Design review of the part built by this model. Coordinates are the model's own, in mm. A direction names the side the tool comes from. Coordinates: 2 decimals unless noted, no trailing zeros. Write each loop counter-clockwise with the first axis right and the second up, starting at its lowest first coordinate (ties: lowest second). Pieces come first, ordered by that corner, then holes. Notation, with made-up numbers: M 81.5,-28.75 L 123.5,-28.75 A35 ccw 123.5,9.25 Z; hole C 81.5,-20 d9. An arc over 180 degrees is marked long. Write item = value, one per line.
```python
from build123d import *

# Parameters (mm, degrees)
ESBO_O1_R                = 15.19
RESSALTO_EXTRUS_O1_DEPTH = 17.37
RESSALTO_EXTRUS_O1_DRAFT = -10
ESBO_O2_R                = 5
CORTE_EXTRUS_O1_DEPTH    = 7
ESBO_O3_R                = 3
CORTE_EXTRUS_O2_DEPTH    = 24.853911629
FILETE1_R                = 2


with BuildPart() as part:
    # Esboço1 → Ressalto-extrusão1 (with draft: the straight prism first)
    with BuildSketch(Plane(origin=(0, 0, 0), x_dir=(1, 0, 0), z_dir=(0, 1, 0))):
        Circle(ESBO_O1_R)
    extrude(amount=-RESSALTO_EXTRUS_O1_DEPTH)
    # Ressalto-extrusão1: the draft: its side faces are tilted about the plane it starts from
    ressalto_extrus_o1_sides = [part.faces().sort_by_distance(p)[0] for p in [
        (-15.19, -8.685, 0),
    ]]
    draft(ressalto_extrus_o1_sides, Plane(origin=(0, 0, 0), x_dir=(1, 0, 0), z_dir=(0, 1, 0)), RESSALTO_EXTRUS_O1_DRAFT)

    # Esboço2 → Corte-extrusão1 (cut)
    with BuildSketch(Plane.XZ.offset(17.37)):
        with Locations(Location((0, 0, 0), (0, 0, 270))):
            Circle(ESBO_O2_R)
    extrude(amount=-CORTE_EXTRUS_O1_DEPTH, mode=Mode.SUBTRACT)

    # Esboço3 → Corte-extrusão2 (cut, through all)
    with BuildSketch(Plane.XZ.offset(10.37)):
        with Locations(Location((0, 0, 0), (0, 0, 270))):
            Circle(ESBO_O3_R)
    extrude(amount=-CORTE_EXTRUS_O2_DEPTH, mode=Mode.SUBTRACT)

    # Filete1
    filete1_edges = [part.edges().sort_by_distance(p)[0] for p in [
        (-12.127200345, -17.37, 0),
    ]]
    fillet(filete1_edges, radius=FILETE1_R)


solid = part.part
```
Q1. Consider section A-A, the plane z = 0. State the section outline as (x, y) points, and give its area (3 significant figures).
Check result:
outline = M -15.19,0 L -12.42,-15.72 A2 ccw -10.45,-17.37 L -5,-17.37 L -5,-10.37 L -3,-10.37 L -3,0 Z; M 3,-10.37 L 5,-10.37 L 5,-17.37 L 10.45,-17.37 A2 ccw 12.42,-15.72 L 15.19,0 L 3,0 Z
area = 341 mm²
Q2. For P1, Ø8, axis at x = 12, y = -15, coming from the -Z side; P2, Ø6, axis at x = -9, z = -10.5, coming from the -Y side; P3, Ø4, axis at x = -6.5, y = -8, coming from the +Z side, all flat-tipped, find the tip position at first contact; note any pin that passes through.
Check result:
P1 = -9.79
P2 = -17.33
P3 = 13.12
Q3. Consider section C-C, the plane y = -14. State the section outline as (x, z) points, and give its area (3 significant figures).
Check result:
outline = C 0,0 d25.44; hole C 0,0 d10
area = 430 mm²
Q4. The part is to be moulded in two halves that separate along Z. For faces 1 (the conical face through (13, -9, -4)), 2 (the flat face through (2, -17.37, -5)), 3 (the cylindrical face through (0.9, -5.26, -2.86)), say which applies: +Z half, -Z half, draft (parallel to the pull), parting line (faces both ways), or undercut.
Check result:
face_1 = parting line
face_2 = draft
face_3 = undercut
Q5. Machinability: for faces 4 (the flat face through (-0.2, 0, 3.2)), 5 (the flat face through (-3.3, -10.37, 0.1)), which of the approach directions +Z, -Z, +X, -X, +Y, -Y give a long, thin tool a straight path to every point of the face, cutting with its end or side? Answer none if there is none.
Check result:
face_4 = +Z, -Z, +X, -X, +Y
face_5 = -Y
Q6. Consider section B-B, the plane y = -9.75. State the section outline as (x, z) points, and give its area (3 significant figures).
Check result:
outline = C 0,0 d26.94; hole C 0,0 d6
area = 542 mm²
Q7. Wall thickness on line 1 (X direction, y = -13.5, z = 0); line 2 (X direction, y = -5, z = 0); line 3 (Z direction, x = 2.5, y = -12): over which ranges is each line inside the solid? List them lowest first.
Check result:
line_1 = -12.81 to -5, 5 to 12.81
line_2 = -14.31 to -3, 3 to 14.31
line_3 = -12.83 to -4.33, 4.33 to 12.83
